```python
from build123d import *

# Parameters (mm, degrees)
SKETCH_R     = 3.373437
PAD_DEPTH    = 9.525
SKETCH001_W  = 12.6492
SKETCH001_H  = 0.254
POCKET_DEPTH = 57.15


with BuildPart() as part:
    # Sketch → Pad (new body)
    with BuildSketch(Plane.XY):
        Polygon((50.8, 0), (0, 0), (0, -127), (114.3, -127), (114.3, -107.95), (50.8, -107.95), align=None)
        with Locations((12.7, -12.7)):
            Circle(SKETCH_R, mode=Mode.SUBTRACT)
        with Locations((38.1, -12.7)):
            Circle(SKETCH_R, mode=Mode.SUBTRACT)
    extrude(amount=PAD_DEPTH)

    # Sketch001 → Pocket (cut)
    with BuildSketch(Plane.YZ.offset(114.3)):
        Polygon((-126.5936, 8.763), (-123.40082, 3.175), (-127, 3.175), (-127, 12.7), (-107.95, 12.7), (-107.95, 3.175), (-111.54918, 3.175), (-108.3564, 8.763), (-108.3564, 9.525), (-111.1504, 9.525), (-111.1504, 9.271), (-123.7996, 9.271), (-123.7996, 9.525), (-126.5936, 9.525), align=None)
        with Locations((-117.475, 0.127)):
            Rectangle(SKETCH001_W, SKETCH001_H)
    extrude(amount=-POCKET_DEPTH, mode=Mode.SUBTRACT)


solid = part.part
```
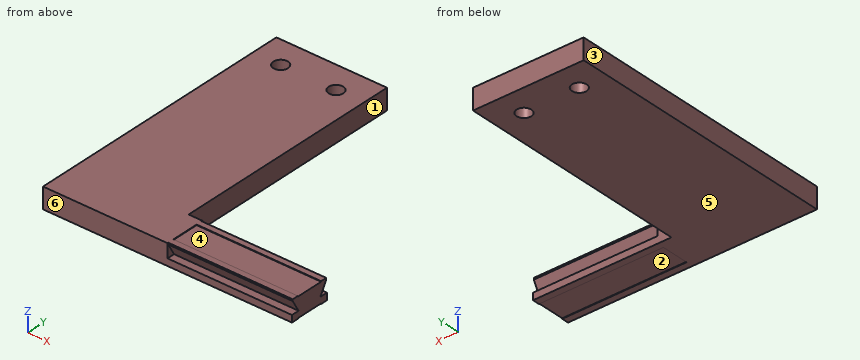
Geometry: final body of the model. Coordinates: model frame, mm. Face numbers are marked on the shaded views. A direction names the side the tool comes from. Coordinates: 2 decimals unless noted, no trailing zeros. Loops run counter-clockwise (first coordinate to the right, second up) from the corner with the lowest first, then second, coordinate; pieces in that order, holes last. Notation, with made-up numbers: M 86.25,89 L 98.25,89 A22 ccw 98.25,107 Z; hole C -18.75,14.25 d4. An arc over 180 degrees is marked long. Put each result on its own line as item: value.
(1) Access query for the marked faces 1, 2 and 3. Directions: +Z, -Z, +X, -X, +Y, -Y. A direction counts if a zero-diameter tool reaches every point of the face in a straight line with its end or side. Return the directions, or none.
Answer sheet:
face 1: +Z, -Z, +X, +Y
face 2: -Z, +X
face 3: +Z, -Z, -X, +Y, -Y
(2) Cut plane B-B on y = -12.7. Return the cut outline in (x, z) (3 decimals), then the cut area to 3 significant figures.
Answer sheet:
outline: M 0,0 L 9.327,0 L 9.327,9.525 L 0,9.525 Z; M 16.073,0 L 34.727,0 L 34.727,9.525 L 16.073,9.525 Z; M 41.473,0 L 50.8,0 L 50.8,9.525 L 41.473,9.525 Z
area: 355 mm^2
(3) Draft query along Y for the marked faces 4, 5 and 6. Return one class per face: pulls with the +Y half, pulls with the -Y half, needs draft (parallel to the pull), parting line crosses it, or undercut.
Answer sheet:
face 4: undercut
face 5: needs draft
face 6: pulls with the -Y half
(4) Material intervals for probe 1 along Y at (x, z) = (38.1, 2.75); probe 2 along X at (y, z) = (-49.5, 7); probe 3 along Y at (x, z) = (56, 2.75), sorted ascending.
Answer sheet:
probe 1: y = -127 to -16.07, -9.33 to 0
probe 2: x = 0 to 50.8
probe 3: y = -127 to -107.95
(5) Cut plane D-D on x = 75.5. Return the cut outline in (y, z) (3 decimals), then the cut area to 3 significant figures.
Answer sheet:
outline: M -127,0 L -123.8,0 L -123.8,0.254 L -111.15,0.254 L -111.15,0 L -107.95,0 L -107.95,3.175 L -111.549,3.175 L -108.356,8.763 L -108.356,9.525 L -111.15,9.525 L -111.15,9.271 L -123.8,9.271 L -123.8,9.525 L -126.594,9.525 L -126.594,8.763 L -123.401,3.175 L -127,3.175 Z
area: 152 mm^2
(6) Cut plane C-C on z = 1.75. Return the cut outline in (x, y).
Answer sheet:
outline: M 0,-127 L 114.3,-127 L 114.3,-107.95 L 50.8,-107.95 L 50.8,0 L 0,0 Z; hole C 12.7,-12.7 d6.75; hole C 38.1,-12.7 d6.75
(7) First-contact query: pin 1 (4 mm diameter, centred on x = 102, z = 4.5, fed in from +Y); pin 2 (5 mm diameter, centred on x = 81, z = 7, fed in from +Y); pin 3 (1.5 mm diameter, centred on y = -44.5, z = 6, fed in from +X); pin 4 (5.5 mm diameter, centred on x = 38.1, y = -12.7, fed in from +Z). Flat tips, straight axial feed; report the tip coordinate or a pass-through.
Answer sheet:
pin 1: stops at y = -107.95
pin 2: stops at y = -108.36
pin 3: stops at x = 50.8
pin 4: passes through
(8) Cut plane A-A on x = 38.1. Return the cut outline in (y, z) (3 decimals), then the cut area to 3 significant figures.
Answer sheet:
outline: M -127,0 L -16.073,0 L -16.073,9.525 L -127,9.525 Z; M -9.327,0 L 0,0 L 0,9.525 L -9.327,9.525 Z
area: 1,150 mm^2
